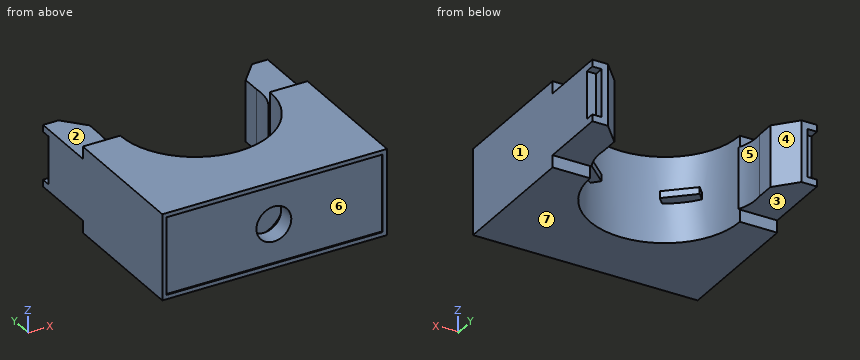
from build123d import *

# Parameters (mm, degrees)
SKETCH1_W               = 41.91
SKETCH1_H               = 38.1
EXTRUDE1_DEPTH          = 16.002
CUT_EXTRUDE1_DEPTH      = 17.002
SKETCH3_W               = 2.27457
SKETCH3_H               = 12.7
CUT_EXTRUDE2_DEPTH      = 21.955
CUT_EXTRUDE2_DEPTH_BACK = 21.955
SKETCH4_W               = 40.3225
SKETCH4_H               = 14.4145
CUT_EXTRUDE3_DEPTH      = 0.254
SKETCH5_W               = 1.731382872
SKETCH5_H               = 8.90143
CUT_EXTRUDE4_DEPTH      = 1.778
EXTRUDE2_DEPTH          = 0.635


with BuildPart() as part:
    # Sketch1 → Extrude1 (new body)
    with BuildSketch(Plane.XY):
        Rectangle(SKETCH1_W, SKETCH1_H)
    extrude(amount=EXTRUDE1_DEPTH)

    # Sketch2 → Cut-Extrude1 (cut, through all)
    with BuildSketch(Plane.XY.offset(16.002)):
        with BuildLine():
            Line((-13.97, 6.35), (-13.6906, 6.35))
            ThreePointArc((-13.6906, 6.35), (-14.51249132, 8.917230674), (-14.5494375, 11.6125625))
            Line((-14.5494375, 11.6125625), (-14.5494375, 15.113))
            Line((-14.5494375, 15.113), (-18.049875, 19.05))
            Line((-18.049875, 19.05), (18.049875, 19.05))
            Line((18.049875, 19.05), (14.5494375, 15.113))
            Line((14.5494375, 15.113), (14.5494375, 11.6125625))
            ThreePointArc((14.5494375, 11.6125625), (14.51249132, 8.917230674), (13.6906, 6.35))
            Line((13.6906, 6.35), (13.97, 6.35))
            ThreePointArc((13.97, 6.35), (0, -7.62), (-13.97, 6.35))
        make_face()
    extrude(amount=-CUT_EXTRUDE1_DEPTH, mode=Mode.SUBTRACT)

    # Sketch3 → Cut-Extrude2 (cut, two sides)
    with BuildSketch(Plane(origin=(0, 0, 0), x_dir=(0, 0, -1), z_dir=(1, 0, 0))) as cut_extrude2_sk:
        with Locations((-14.864715, 12.7)):
            Rectangle(SKETCH3_W, SKETCH3_H)
        with Locations((-1.137285, 12.7)):
            Rectangle(SKETCH3_W, SKETCH3_H)
    extrude(amount=CUT_EXTRUDE2_DEPTH, mode=Mode.SUBTRACT)
    extrude(cut_extrude2_sk.sketch, amount=-CUT_EXTRUDE2_DEPTH_BACK, mode=Mode.SUBTRACT)

    # Sketch4 → Cut-Extrude3 (cut)
    with BuildSketch(Plane.XZ.offset(19.05)):
        with Locations((0, 8.001)):
            Rectangle(SKETCH4_W, SKETCH4_H)
    extrude(amount=-CUT_EXTRUDE3_DEPTH, mode=Mode.SUBTRACT)

    # Sketch5 → Cut-Extrude4 (cut)
    with BuildSketch(Plane(origin=(0, 19.05, 0), x_dir=(1, 0, 0), z_dir=(0, 1, 0))):
        with Locations((-20.089308564, -8.001)):
            Rectangle(SKETCH5_W, SKETCH5_H)
        with Locations((20.089308564, -8.001)):
            Rectangle(SKETCH5_W, SKETCH5_H)
    extrude(amount=-CUT_EXTRUDE4_DEPTH, mode=Mode.SUBTRACT)

    # Sketch6 → Cut-Revolve1 (revolve, cut)
    with BuildSketch(Plane(origin=(0, 0, 8.001), x_dir=(-1, 0, 0), z_dir=(0, 0, -1)), mode=Mode.PRIVATE) as cut_revolve1_sk:
        Polygon((3.25, -18.796), (0, -18.796), (0, -12.296), (5.842, -12.296), (5.842, -15.546), (3.25, -15.546), align=None)
    revolve(cut_revolve1_sk.sketch.rotate(Axis((0, 0, 8.001), (0, -1, 0)), 270), axis=Axis((0, 0, 8.001), (0, -1, 0)), mode=Mode.SUBTRACT)  # turned: the seam where the file's is

    # Sketch7 → Extrude2 (add, symmetric)
    with BuildSketch(Plane(origin=(0, 0, 8.001), x_dir=(-1, 0, 0), z_dir=(0, 0, -1))):
        with BuildLine():
            Line((5.443056808, -4.606163762), (10.327190387, -0.208470134))
            Line((10.327190387, -0.208470134), (11.527527053, -1.541579058))
            ThreePointArc((11.527527053, -1.541579058), (9.347754571, -4.031733212), (6.643393474, -5.939272686))
            Line((6.643393474, -5.939272686), (5.443056808, -4.606163762))
        make_face()
        with BuildLine():
            Line((-5.443056808, -4.606163762), (-6.643393474, -5.939272686))
            ThreePointArc((-6.643393474, -5.939272686), (-9.347754571, -4.031733212), (-11.527527053, -1.541579058))
            Line((-11.527527053, -1.541579058), (-10.327190387, -0.208470134))
            Line((-10.327190387, -0.208470134), (-5.443056808, -4.606163762))
        make_face()
    extrude(amount=EXTRUDE2_DEPTH, both=True)


solid = part.part
Could you check a few things on this model? Use its own coordinates, in mm. Face numbers are marked on the shaded views. A direction names the side the tool comes from. Round coordinates to 2 decimals unless told otherwise and drop trailing zeros. Order: outer loops, then holes, each group sorted by start corner. A loop starts at its lowest first (then second) coordinate and runs counter-clockwise, first axis right, second up.
Q1. Imagine slicing it at D-D, the plane y = 16. List the corners of the cut face in (x, z) for me (3 decimals).
Geometry says:
outline: (-20.955, 2.275) - (-15.338, 2.275) - (-15.338, 13.727) - (-20.955, 13.727) - close; (15.338, 2.275) - (20.955, 2.275) - (20.955, 13.727) - (15.338, 13.727) - close
Q2. Thinking about a two-plate mould opening in Y: for the marked faces 5, 6 and 7, which applies, released by +Y, released by -Y, zero draft, split by the parting line, or undercut?
Geometry says:
face 5: undercut
face 6: released by -Y
face 7: zero draft
Q3. Imagine slicing it at B-B, the plane x = 0. List the corners of the cut face in (y, z) for me, then the cut area to 3 significant figures.
Geometry says:
outline: (-19.05, 0) - (-7.62, 0) - (-7.62, 16) - (-19.05, 16) - (-19.05, 15.21) - (-18.8, 15.21) - (-18.8, 11.25) - (-15.55, 11.25) - (-15.55, 13.84) - (-12.3, 13.84) - (-12.3, 2.16) - (-15.55, 2.16) - (-15.55, 4.75) - (-18.8, 4.75) - (-18.8, 0.79) - (-19.05, 0.79) - close
area: 120 mm2
Q4. Which directions (+Z, -Z, +X, -X, +Y, -Y) give clear straight access to the entire face, cutting with the end or side of a thin tool? Please do the marked faces 1, 2, 3 and 4.
Geometry says:
face 1: +Z, -Z, +X, +Y, -Y
face 2: +Z, +X, -X, +Y
face 3: -Z, +X, -X, +Y
face 4: +Z, -Z, +Y
Q5. Imagine slicing it at A-A, the plane y = -4. List the corners of the cut face in (x, z) for me (3 decimals).
Geometry says:
outline: (-20.955, 0) - (-9.383, 0) - (-9.383, 7.366) - (-6.116, 7.366) - (-6.116, 8.636) - (-9.383, 8.636) - (-9.383, 16.002) - (-20.955, 16.002) - close; (6.116, 7.366) - (9.383, 7.366) - (9.383, 0) - (20.955, 0) - (20.955, 16.002) - (9.383, 16.002) - (9.383, 8.636) - (6.116, 8.636) - close
Q6. Please list where these lines run through material, in increasing order: probe 1 along X at (y, z) = (12.5, 4.25) (3 decimals); probe 2 along Y at (x, z) = (3.5, 9.5); probe 3 along X at (y, z) = (-2, 9) (3 decimals).
Geometry says:
probe 1: x = -20.955 to -14.549, 14.549 to 20.955
probe 2: y = -18.8 to -15.55, -12.3 to -7.17
probe 3: x = -20.955 to -11.2, 11.2 to 20.955
Q7. I'm going to push flat-ended pins straight in: P1, Ø8, axis at x = -16, y = 11, coming from the +Z side; P2, Ø1.5, axis at x = 16, y = 11, coming from the -Z side; P3, Ø1.4, axis at x = 20.5, z = 9, coming from the +Y side; P4, Ø6, axis at x = 7, y = -15, coming from the -Z side. Where does each tip first touch, or does it pass through?
Geometry says:
P1: stops at z = 13.73
P2: stops at z = 2.27
P3: stops at y = 17.27
P4: stops at z = 0
